Geometry: final body of the model. Coordinates: model frame, mm. A direction names the side the tool comes from. Coordinates: 2 decimals unless noted, no trailing zeros. Order: outer loops, then holes, each group sorted by start corner. A loop starts at its lowest first (then second) coordinate and runs counter-clockwise, first axis right, second up. Notation, with made-up numbers: (0.5, -27) - (42.5, -27) arc R29 ccw to (42.5, 2) - close; hole circle Ø11 at (-36.75, 21). An arc over 180 degrees is marked (long way). Use a Markdown table: item, result. Add a question column.
```python
from build123d import *

# Parameters (mm, degrees)
SKETCH1_W         = 19.05
SKETCH1_H         = 8.636
HOLE1_D           = 3.9624
HOLE1_DEPTH       = 8.636
HOLE1_CBORE_D     = 5.969
HOLE1_CBORE_DEPTH = 3.7592
HOLE2_D           = 3.9624
HOLE2_DEPTH       = 8.636
HOLE2_CBORE_D     = 5.969
HOLE2_CBORE_DEPTH = 3.7592
HOLE3_D           = 3.9624
HOLE3_DEPTH       = 8.636
HOLE3_CBORE_D     = 5.969
HOLE3_CBORE_DEPTH = 3.7592
HOLE4_D           = 3.9624
HOLE4_DEPTH       = 8.636
HOLE4_CBORE_D     = 5.969
HOLE4_CBORE_DEPTH = 3.7592
HOLE5_D           = 20.6248
HOLE5_DEPTH       = 4.318
HOLE6_D           = 3.4544
HOLE6_DEPTH       = 4.318
HOLE7_D           = 3.4544
HOLE7_DEPTH       = 4.318
HOLE8_D           = 3.4544
HOLE8_DEPTH       = 4.318
HOLE9_D           = 3.4544
HOLE9_DEPTH       = 4.318


with BuildPart() as part:
    # Sketch1 → Revolve1 (revolve)
    with BuildSketch(Plane.XY):
        with Locations((9.525, 4.318)):
            Rectangle(SKETCH1_W, SKETCH1_H)
    revolve(axis=Axis((0, 0, 0), (0, 1, 0)))

    # Sketch2 → Cut-Revolve1 (revolve, cut)
    with BuildSketch(Plane.XY):
        Polygon((-19.05, 5.08), (-19.05, 9.04875), (-18.542, 9.04875), (-18.542, 7.493), (-18.11274, 7.06374), (-7.874, 7.06374), (-6.728687177, 5.08), align=None)
    revolve(axis=Axis((-6.728687177, 5.08, 0), (-1, 0, 0)), mode=Mode.SUBTRACT)

    # Hole1
    with Locations(Plane(origin=(0, 8.636, 0), x_dir=(1, 0, 0), z_dir=(0, 1, 0))):
        with Locations((-10.566882591, -11.331594253)):
            CounterBoreHole(HOLE1_D / 2, HOLE1_CBORE_D / 2, HOLE1_CBORE_DEPTH, depth=HOLE1_DEPTH)

    # Hole2
    with Locations(Plane(origin=(0, 8.636, 0), x_dir=(1, 0, 0), z_dir=(0, 1, 0))):
        with Locations((11.331594253, -10.566882591)):
            CounterBoreHole(HOLE2_D / 2, HOLE2_CBORE_D / 2, HOLE2_CBORE_DEPTH, depth=HOLE2_DEPTH)

    # Hole3
    with Locations(Plane(origin=(0, 8.636, 0), x_dir=(1, 0, 0), z_dir=(0, 1, 0))):
        with Locations((10.566882591, 11.331594253)):
            CounterBoreHole(HOLE3_D / 2, HOLE3_CBORE_D / 2, HOLE3_CBORE_DEPTH, depth=HOLE3_DEPTH)

    # Hole4
    with Locations(Plane(origin=(0, 8.636, 0), x_dir=(1, 0, 0), z_dir=(0, 1, 0))):
        with Locations((-11.331594253, 10.566882591)):
            CounterBoreHole(HOLE4_D / 2, HOLE4_CBORE_D / 2, HOLE4_CBORE_DEPTH, depth=HOLE4_DEPTH)

    # Hole5
    with Locations(Plane(origin=(0, 0, 0), x_dir=(-1, 0, 0), z_dir=(0, -1, 0))):
        with Locations((0, 0)):
            Hole(HOLE5_D / 2, depth=HOLE5_DEPTH)

    # Hole6
    with Locations(Plane(origin=(0, 0, 0), x_dir=(-1, 0, 0), z_dir=(0, -1, 0))):
        with Locations((14.930490242, -4.140591399)):
            Hole(HOLE6_D / 2, depth=HOLE6_DEPTH)

    # Hole7
    with Locations(Plane(origin=(0, 0, 0), x_dir=(-1, 0, 0), z_dir=(0, -1, 0))):
        with Locations((-4.140591399, -14.930490242)):
            Hole(HOLE7_D / 2, depth=HOLE7_DEPTH)

    # Hole8
    with Locations(Plane(origin=(0, 0, 0), x_dir=(-1, 0, 0), z_dir=(0, -1, 0))):
        with Locations((-14.930490242, 4.140591399)):
            Hole(HOLE8_D / 2, depth=HOLE8_DEPTH)

    # Hole9
    with Locations(Plane(origin=(0, 0, 0), x_dir=(-1, 0, 0), z_dir=(0, -1, 0))):
        with Locations((4.140591399, 14.930490242)):
            Hole(HOLE9_D / 2, depth=HOLE9_DEPTH)


solid = part.part
```
1) Access query for faces 1 (the cylindrical face through (-18.736, 1.114, -0.149)), 2 (the flat face through (15, 4.318, -4)), 3 (the cylindrical face through (11.94, 6.78, -8.68)), 4 (the flat face through (0, 8.636, 0)). Directions: +Z, -Z, +X, -X, +Y, -Y. A direction counts if a zero-diameter tool reaches every point of the face in a straight line with its end or side. Return the directions, or none.
2) Section query B-B (x = 11). Return the cut outline in (y, z), and give its area (3 significant figures).
3) Section query D-D (z = -15.5). Return the cut outline in (x, y).
4) First-contact query: pin 1 (3 mm diameter, centred on y = 5.5, z = -12.5, fed in from +X); pin 2 (4 mm diameter, centred on y = 7.5, z = -14, fed in from +X); pin 3 (3 mm diameter, centred on x = -12, z = -10.5, fed in from +Y); pin 4 (3 mm diameter, centred on x = 10.57, z = -11.33, fed in from -Y). Flat tips, straight axial feed; report the tip coordinate or a pass-through.
5) Line query: line 1 (Z direction, x = -3, y = 2.5); line 2 (Z direction, x = 11.5, y = 5); line 3 (Y direction, x = 3, z = -8). Output: solid intervals per line, ascending. Write a range as from..to.
6) Section query C-C (x = 0). Return the cut outline in (y, z), and give its area (3 significant figures).
7) Draft query along Y for faces 5 (the flat face through (-9, 4.877, -10)), 6 (the conical face through (-6.91, 5.38, -0.1)), 7 (the cylindrical face through (-11.72, 6.783, -13.526)). Return one class per face: released by +Y, released by -Y, zero draft, split by the parting line, or undercut.
8) Section query A-A (x = -12). Return the cut outline in (y, z), and give its area (3 significant figures).
From the geometry:
| question | item | result |
|---|---|---|
| 1 | face 1 | -X |
| 1 | face 2 | -Y |
| 1 | face 3 | +Y |
| 1 | face 4 | +Z, -Z, +X, -X, +Y |
| 2 | outline | (0, -15.55) - (8.64, -15.55) - (8.64, -14.28) - (4.88, -14.28) - (4.88, -13.26) - (0, -13.26) - close; (0, -9.4) - (4.88, -9.4) - (4.88, -8.38) - (8.64, -8.38) - (8.64, 7.6) - (4.88, 7.6) - (4.88, 8.61) - (0, 8.61) - close; (0, 12.52) - (4.88, 12.52) - (4.88, 13.53) - (8.64, 13.53) - (8.64, 15.55) - (0, 15.55) - close |
| 2 | area | 186 mm^2 |
| 3 | outline | (-11.07, 0) - (-5.77, 0) - (-5.77, 4.32) - (-2.51, 4.32) - (-2.51, 0) - (11.07, 0) - (11.07, 8.64) - (-11.07, 8.64) - close |
| 4 | pin 1 | stops at x = 15.55 |
| 4 | pin 2 | stops at x = 14.8 |
| 4 | pin 3 | stops at y = 4.88 |
| 4 | pin 4 | passes through |
| 5 | line 1 | z = -18.81..-16.23, -13.63..-9.87, 9.87..18.81 |
| 5 | line 2 | z = -15.19..-14.17, -8.5..7.59, 13.55..15.19 |
| 5 | line 3 | y = 4.32..8.64 |
| 6 | outline | (0, -19.05) - (8.64, -19.05) - (8.64, 19.05) - (0, 19.05) - (0, 10.31) - (4.32, 10.31) - (4.32, -10.31) - (0, -10.31) - close |
| 6 | area | 240 mm^2 |
| 7 | face 5 | released by +Y |
| 7 | face 6 | undercut |
| 7 | face 7 | zero draft |
| 8 | outline | (0, -14.8) - (8.64, -14.8) - (8.64, -13.48) - (4.88, -13.48) - (4.88, -12.43) - (0, -12.43) - close; (0, -8.7) - (4.88, -8.7) - (4.88, -7.66) - (8.64, -7.66) - (8.64, 8.71) - (4.88, 8.71) - (4.88, 9.96) - (0, 9.96) - close; (0, 12.7) - (4.88, 12.7) - (4.88, 13.95) - (8.64, 13.95) - (8.64, 14.8) - (0, 14.8) - close; hole circle Ø3.97 at (5.08, 0) |
| 8 | area | 170 mm^2 |
